Part model, mm, in its own coordinate system. A direction names the side the tool comes from. Round coordinates to 2 decimals unless told otherwise and drop trailing zeros. Order: outer loops, then holes, each group sorted by start corner. A loop starts at its lowest first (then second) coordinate and runs counter-clockwise, first axis right, second up. Notation, with made-up numbers: (45, 23.25) - (99, 23.25) arc R36 ccw to (99, 57.25) - close; hole circle Ø8 at (-9.75, 78). An arc over 180 degrees is marked (long way). Answer as a JSON object with one key per item and string values.
```python
from build123d import *

# Parameters (mm, degrees)
SKETCH1_W           = 60
SKETCH1_H           = 210
BOSS_EXTRUDE1_DEPTH = 5
SKETCH2_W           = 3.1
SKETCH2_H           = 20
CUT_EXTRUDE1_DEPTH  = 5
SKETCH3_R           = 1.65
CUT_EXTRUDE2_DEPTH  = 5


with BuildPart() as part:
    # Sketch1 → Boss-Extrude1 (new body)
    with BuildSketch(Plane(origin=(0, 0, 0), x_dir=(1, 0, 0), z_dir=(0, 1, 0))):
        with Locations((30, 105)):
            Rectangle(SKETCH1_W, SKETCH1_H)
    extrude(amount=BOSS_EXTRUDE1_DEPTH)

    # Sketch2 → Cut-Extrude1 (cut)
    with BuildSketch(Plane(origin=(0, 5, 0), x_dir=(1, 0, 0), z_dir=(0, 1, 0))):
        with Locations((48.45, 40)):
            Rectangle(SKETCH2_W, SKETCH2_H)
        with Locations((40.35, 40)):
            Rectangle(SKETCH2_W, SKETCH2_H)
    extrude(amount=-CUT_EXTRUDE1_DEPTH, mode=Mode.SUBTRACT)

    # Sketch3 → Cut-Extrude2 (cut)
    with BuildSketch(Plane(origin=(0, 5, 0), x_dir=(1, 0, 0), z_dir=(0, 1, 0))):
        with Locations(Location((55, 180, 0), (0, 0, 270))):
            Circle(SKETCH3_R)
        with Locations(Location((55, 124, 0), (0, 0, 90))):
            Circle(SKETCH3_R)
        with Locations(Location((31, 124, 0), (0, 0, 270))):
            Circle(SKETCH3_R)
        with Locations(Location((31, 180, 0), (0, 0, 90))):
            Circle(SKETCH3_R)
    extrude(amount=-CUT_EXTRUDE2_DEPTH, mode=Mode.SUBTRACT)


solid = part.part
```
Item 1: Two-plate mould, pull along X, no slides. Class faces 1 (the flat face through (60, 2, -104)), 2 (the flat face through (0, 2, -104)), 3 (the flat face through (46.9, 3, -40)), 4 (the flat face through (30, 2, -210)): pulls with the +X half, pulls with the -X half, needs draft (parallel to the pull), parting line crosses it, or undercut.
Taken from the geometry:
{"face 1": "pulls with the +X half", "face 2": "pulls with the -X half", "face 3": "undercut", "face 4": "needs draft"}
Item 2: Tool access for faces 5 (the flat face through (50, 3, -40)), 6 (the flat face through (30, 2, 0)): list every direction of +Z, -Z, +X, -X, +Y, -Y with a clear straight run to the whole face (end or side of a thin tool).
Taken from the geometry:
{"face 5": "+Y, -Y", "face 6": "+Z, +X, -X, +Y, -Y"}
Item 3: Drop flat-ended pins along their axis: P1, Ø1.5, axis at y = 3, z = -38, coming from the -X side; P2, Ø2.5, axis at x = 55, z = -180, coming from the -Y side. Give the stop position or say it passes through.
Taken from the geometry:
{"P1": "x = 0", "P2": "through"}
Item 4: Cut at A-A (z = -40). Write the cut outline in (x, y).
Taken from the geometry:
{"outline": "(0, 0) - (38.8, 0) - (38.8, 5) - (0, 5) - close; (41.9, 0) - (46.9, 0) - (46.9, 5) - (41.9, 5) - close; (50, 0) - (60, 0) - (60, 5) - (50, 5) - close"}
Item 5: Probe L1, parallel to X at y = 3.55, z = -180; L2, parallel to X at y = 0.45, z = -45.5; L3, parallel to Z at x = 49.5, y = 3.95. List the from-to ranges inside material, lowest first. Write a range as from..to.
Taken from the geometry:
{"L1": "0..29.35, 32.65..53.35, 56.65..60", "L2": "0..38.8, 41.9..46.9, 50..60", "L3": "-210..-50, -30..0"}
